from build123d import *


with BuildPart() as part:
    # По траектории4: sweep along a curve in space
    with BuildLine() as sweep_4_path:
        Line((-460.4, 69.25, 0), (-460.4, 4, 0))
        Line((-460.4, 4, 0), (0, 4, 0))
    # Эскиз2<3> → По траектории4 (sweep)
    with BuildSketch(Plane.XZ.offset(-69.25)):
        with BuildLine():
            Line((-460.4, -25), (-460.4, 25))
            Line((-460.4, 25), (-428.4, 25))
            Line((-428.4, 25), (-428.4, 23.1))
            ThreePointArc((-428.4, 23.1), (-429.132233047, 21.332233047), (-430.9, 20.6))
            Line((-430.9, 20.6), (-450, 20.6))
            ThreePointArc((-450, 20.6), (-454.242640687, 18.842640687), (-456, 14.6))
            Line((-456, 14.6), (-456, -14.6))
            ThreePointArc((-456, -14.6), (-454.242640687, -18.842640687), (-450, -20.6))
            Line((-450, -20.6), (-430.9, -20.6))
            ThreePointArc((-430.9, -20.6), (-429.132233047, -21.332233047), (-428.4, -23.1))
            Line((-428.4, -23.1), (-428.4, -25))
            Line((-428.4, -25), (-460.4, -25))
        make_face()
    sweep(path=sweep_4_path.line, transition=Transition.RIGHT)

    # Зеркальное отражение2: part across plane


with BuildPart() as part_1:
    add(part.part)
    add(part.part.mirror(Plane(origin=(0, 33.5, 23.1), x_dir=(0, 0, 1), z_dir=(-1, 0, 0))))


solid = part_1.part
Model file for the job. Use its own axes, mm. A direction names the side the tool comes from. Round coordinates to 2 decimals unless told otherwise and drop trailing zeros. Order: outer loops, then holes, each group sorted by start corner. A loop starts at its lowest first (then second) coordinate and runs counter-clockwise, first axis right, second up. Notation, with made-up numbers: M -29,-26 L -19,-26 A21 cw -19,1 Z; hole C -14,68 d3. An arc over 180 degrees is marked long. Write each question's results on one line, items separated by ' | '. Start each with the question number.
(1) Which spindle directions (+Z, -Z, +X, -X, +Y, -Y) get a long thin tool onto all of the face, cutting with end or side? Do faces 1 (the face through (456.2, 69.25, 2)), 2 (the face through (2, 27, 20.6)). Say none if no direction does.
(2) Saw through at B-B, the plane z = -3.5. Give the cut face in (x, y), then the cut area to 3 significant figures.
(3) Two-plate mould, pull along X, no slides. Class faces 3 (the face through (-460.4, 36, 0)), 4 (the face through (-6, 14, 25)), 5 (the face through (-456, 38, 0)): pulls with the +X half, pulls with the -X half, needs draft (parallel to the pull), parting line crosses it, or undercut.
(4) Saw through at C-C, the plane x = -246. Give the cut face in (y, z), then the cut area to 3 significant figures.
(5) Saw through at A-A, the plane y = 54.5. Give the cut face in (x, z).
(6) Probe probe 1 along X at (y, z) = (56.5, -23); probe 2 along Z at (x, y) = (91, 20); probe 3 along X at (y, z) = (49, 11). List the from-to ranges inside material, lowest first. Write a range as from..to.
(7) Drop flat-ended pins along their axis: pin 1 (0.6 mm diameter, centred on x = -169.5, z = -23.5, fed in from +Y); pin 2 (10 mm diameter, centred on x = -329.5, z = 0, fed in from +Y); pin 3 (8 mm diameter, centred on x = -0.5, z = 12, fed in from +Y). Give the stop position or say it passes through.
Established:
1) face 1: +Z, -Z, +X, -X, +Y | face 2: +Y
2) outline: M -460.4,4 L 460.4,4 L 460.4,69.25 L 456,69.25 L 456,8.4 L -456,8.4 L -456,69.25 L -460.4,69.25 Z | area: 4,590 mm^2
3) face 3: pulls with the -X half | face 4: needs draft | face 5: undercut
4) outline: M 4,-25 L 36,-25 L 36,-23.1 A2.5 ccw 33.5,-20.6 L 14.4,-20.6 A6 cw 8.4,-14.6 L 8.4,14.6 A6 cw 14.4,20.6 L 33.5,20.6 A2.5 ccw 36,23.1 L 36,25 L 4,25 Z | area: 476 mm^2
5) outline: M -460.4,-25 L -428.4,-25 L -428.4,-23.1 A2.5 ccw -430.9,-20.6 L -450,-20.6 A6 cw -456,-14.6 L -456,14.6 A6 cw -450,20.6 L -430.9,20.6 A2.5 ccw -428.4,23.1 L -428.4,25 L -460.4,25 Z; M 428.4,-25 L 460.4,-25 L 460.4,25 L 428.4,25 L 428.4,23.1 A2.5 ccw 430.9,20.6 L 450,20.6 A6 cw 456,14.6 L 456,-14.6 A6 cw 450,-20.6 L 430.9,-20.6 A2.5 ccw 428.4,-23.1 Z
6) probe 1: x = -460.4..-428.4, 428.4..460.4 | probe 2: z = -25..-20.6, 20.6..25 | probe 3: x = -460.4..-456, 456..460.4
7) pin 1: stops at y = 36 | pin 2: stops at y = 8.4 | pin 3: stops at y = 8.57
